from build123d import *

# Parameters (mm, degrees)
SKETCH1_W           = 24
SKETCH1_H           = 32.05
SKETCH1_R           = 2.15
BOSS_EXTRUDE1_DEPTH = 37
SKETCH2_R           = 2.15
BOSS_EXTRUDE2_DEPTH = 30
SKETCH3_R           = 3.4
CUT_EXTRUDE1_DEPTH  = 12
FILLET1_R           = 5
SKETCH4_R           = 2.75
BOSS_EXTRUDE3_DEPTH = 5
FILLET2_R           = 1.5


with BuildPart() as part:
    # Sketch1 → Boss-Extrude1 (new body)
    with BuildSketch(Plane(origin=(0, 0, 0), x_dir=(1, 0, 0), z_dir=(0, 1, 0))):
        with Locations((10.056177559, 9.020502124)):
            Rectangle(SKETCH1_W, SKETCH1_H)
        with Locations((5.056177559, 9.020502124)):
            Circle(SKETCH1_R, mode=Mode.SUBTRACT)
        with Locations((15.056177559, 9.020502124)):
            Circle(SKETCH1_R, mode=Mode.SUBTRACT)
        with Locations((10.056177559, 19.895502124)):
            Circle(SKETCH1_R, mode=Mode.SUBTRACT)
        with Locations((10.056177559, -1.854497876)):
            Circle(SKETCH1_R, mode=Mode.SUBTRACT)
    extrude(amount=BOSS_EXTRUDE1_DEPTH)

    # Sketch2 → Boss-Extrude2 (add)
    with BuildSketch(Plane(origin=(0, 37, 0), x_dir=(1, 0, 0), z_dir=(0, 1, 0))):
        with Locations((10.056177559, 19.895502124)):
            Circle(SKETCH2_R)
        with Locations((15.056177559, 9.020502124)):
            Circle(SKETCH2_R)
        with Locations((10.056177559, -1.854497876)):
            Circle(SKETCH2_R)
        with Locations((5.056177559, 9.020502124)):
            Circle(SKETCH2_R)
    extrude(amount=-BOSS_EXTRUDE2_DEPTH)

    # Sketch3 → Cut-Extrude1 (cut)
    with BuildSketch(Plane(origin=(0, 37, 0), x_dir=(1, 0, 0), z_dir=(0, 1, 0))):
        with Locations((10.056177559, 9.020502124)):
            Circle(SKETCH3_R)
    extrude(amount=-CUT_EXTRUDE1_DEPTH, mode=Mode.SUBTRACT)

    # Fillet1
    fillet1_edges = [part.edges().sort_by_distance(p)[0] for p in [
        (22.056177559, 37, -9.020502124),
        (10.056177559, 37, -25.045502124),
        (-1.943822441, 37, -9.020502124),
        (-1.943822441, 18.5, -25.045502124),
        (22.056177559, 18.5, -25.045502124),
        (22.056177559, 18.5, 7.004497876),
        (-1.943822441, 18.5, 7.004497876),
        (10.056177559, 37, 7.004497876),
    ]]
    fillet(fillet1_edges, radius=FILLET1_R)

    # Sketch4 → Boss-Extrude3 (add)
    with BuildSketch(Plane.ZY.offset(1.943822441)):
        with Locations((-9.020502124, 4)):
            Circle(SKETCH4_R)
    extrude(amount=BOSS_EXTRUDE3_DEPTH)

    # Fillet2
    fillet2_edges = [part.edges().sort_by_distance(p)[0] for p in [
        (-6.943822441, 4, -11.770502124),
    ]]
    fillet(fillet2_edges, radius=FILLET2_R)


solid = part.part
The listing builds one solid part. Answer for the finished solid, in the listing's coordinates (mm). A direction names the side the tool comes from. Coordinates: 2 decimals unless noted, no trailing zeros. Order: outer loops, then holes, each group sorted by start corner. A loop starts at its lowest first (then second) coordinate and runs counter-clockwise, first axis right, second up. Notation, with made-up numbers: (-38, 9.25) -> (-13, 9.25) arc R22 ccw to (-13, 18.25) -> close; hole circle Ø6 at (6, 48.5). An arc over 180 degrees is marked (long way). Answer in a Markdown table with one row per item. Add a question column.
Item 1: Which of the six approach directions +Z, -Z, +X, -X, +Y, -Y give full straight-line access (tool end or side, diameter ignored) to faces 4 (the face through (22.056, 16, -9)), 5 (the face through (-3.669, 2.327, -11.203)), 6 (the face through (12.91, 3.45, -9.12))?
Item 2: Find section B-B (z = -13.5). Write down the section's boundary in (x, y), then the cut area to 3 significant figures.
Item 3: Find section C-C (y = 15.5). Write down the section's boundary in (x, z), then the cut area to 3 significant figures.
Item 4: Find the intervals of material crossed by L1, parallel to X at y = 2, z = 1; L2, parallel to X at y = 24, z = -14; L3, parallel to Z at x = 15.75, y = 3.5, in increasing order. Write a range as from..to.
Item 5: Find section A-A (y = 34). Write down the section's boundary in (x, z), then the cut area to 3 significant figures.
Item 6: Determine the mould class of faces 1 (the face through (10, 16, -25.046)), 2 (the face through (10, 25, -9)), 3 (the face through (-0.52, 16.22, 5.5)) for opening direction Z: +Z half, -Z half, draft (parallel to the pull), parting line (faces both ways), or undercut.
Item 7: Find section D-D (x = -4.25). Write down the section's boundary in (y, z).
Item 8: Each of these flat-tipped pins is pushed along its axis until it touches: P1, Ø2, axis at x = 10, z = -7.5, coming from the +Y side; P2, Ø2, axis at x = 6, z = -9.5, coming from the -Y side; P3, Ø8, axis at y = 29.5, z = 1, coming from the -X side. Where does it stop, or does it pass through?
Result set:
| question | item | result |
|---|---|---|
| 1 | face 4 | +Z, -Z, +X, +Y, -Y |
| 1 | face 5 | -X |
| 1 | face 6 | -Y |
| 2 | outline | (-1.94, 0) -> (22.06, 0) -> (22.06, 32) arc R5 ccw to (17.06, 37) -> (3.06, 37) arc R5 ccw to (-1.94, 32) -> close |
| 2 | area | 877 mm² |
| 3 | outline | (-1.94, -20.05) arc R5 ccw to (3.06, -25.05) -> (17.06, -25.05) arc R5 ccw to (22.06, -20.05) -> (22.06, 2) arc R5 ccw to (17.06, 7) -> (3.06, 7) arc R5 ccw to (-1.94, 2) -> close |
| 3 | area | 748 mm² |
| 4 | L1 | x = -1.94..8.08, 12.03..22.06 |
| 4 | L2 | x = -1.94..22.06 |
| 4 | L3 | z = -25.05..-11.06, -6.99..7 |
| 5 | outline | (-1.53, -20.05) arc R4.58 ccw to (3.06, -24.63) -> (17.06, -24.63) arc R4.58 ccw to (21.64, -20.05) -> (21.64, 2) arc R4.58 ccw to (17.06, 6.59) -> (3.06, 6.59) arc R4.58 ccw to (-1.53, 2) -> close; hole circle Ø6.8 at (10.06, -9.02) |
| 5 | area | 669 mm² |
| 6 | face 1 | -Z half |
| 6 | face 2 | undercut |
| 6 | face 3 | +Z half |
| 7 | outline | circle Ø5.5 at (4, -9.02) |
| 8 | P1 | stops at y = 25 |
| 8 | P2 | stops at y = 7 |
| 8 | P3 | stops at x = -1.94 |
